Model file for the job. Use its own axes, mm. A direction names the side the tool comes from. Give positions to 0.01 mm unless a question says otherwise; leave off trailing zeros. Loops run counter-clockwise (first coordinate to the right, second up) from the corner with the lowest first, then second, coordinate; pieces in that order, holes last. Notation, with made-up numbers: M 66.5,37 L 76.5,37 A21 ccw 76.5,49 Z; hole C 17.25,25.5 d7. An arc over 180 degrees is marked long. Use CSV: the item, a comma, the result in double quotes. Start each with the question number.
(1) Slice it at C-C on y = 6. State how many separate pieces and enclosed holes the cut face has, and give its area (3 significant figures).
(2) Slice it at B-B on x = 102.5. List the corners of the cut face in (y, z).
(3) Tool access for faces 3 (the face through (-140, 6, 289.5)), 4 (the face through (-2, 6, 337.5)): list every direction of +Z, -Z, +X, -X, +Y, -Y with a clear straight run to the whole face (end or side of a thin tool).
(4) Two-plate mould, pull along X, no slides. Class faces 1 (the face through (72, 6, -6)), 2 (the face through (-24, 12, -2)): pulls with the +X half, pulls with the -X half, needs draft (parallel to the pull), parting line crosses it, or undercut.
(5) Wall check: line 1 along Z through (x, y) = (-47, 7.5); line 2 along X through (y, z) = (8.75, -297.5); line 3 along X through (y, z) = (9, 129). Give the ranges that are in metal, low to high. Write a range as from..to.
(6) Slice it at A-A on z = -281. List the corners of the cut face in (x, y), and give its area (3 significant figures).
```python
from build123d import *

# Parameters (mm, degrees)
SKETCH1_W               = 310
SKETCH1_H               = 675
SKETCH1_W_2             = 300
SKETCH1_H_2             = 665
SKETCH1_W_3             = 260
SKETCH1_H_3             = 625
SKETCH1_W_4             = 250
SKETCH1_H_4             = 615
BOSS_EXTRUDE1_DEPTH     = 12
SKETCH2_W               = 12
SKETCH2_H               = 12
CUT_EXTRUDE1_DEPTH      = 1
CUT_EXTRUDE1_DEPTH_BACK = 13
SKETCH3_W               = 105
SKETCH3_H               = 12
BOSS_EXTRUDE2_DEPTH     = 12


with BuildPart() as part:
    # Sketch1 → Boss-Extrude1 (new body)
    with BuildSketch(Plane(origin=(0, 0, 0), x_dir=(1, 0, 0), z_dir=(0, 1, 0))):
        Rectangle(SKETCH1_W, SKETCH1_H)
        Rectangle(SKETCH1_W_2, SKETCH1_H_2, mode=Mode.SUBTRACT)
        Rectangle(SKETCH1_W_2, SKETCH1_H_2)
        Rectangle(SKETCH1_W_3, SKETCH1_H_3, mode=Mode.SUBTRACT)
        Rectangle(SKETCH1_W_3, SKETCH1_H_3)
        Rectangle(SKETCH1_W_4, SKETCH1_H_4, mode=Mode.SUBTRACT)
    extrude(amount=BOSS_EXTRUDE1_DEPTH)

    # Sketch2 → Cut-Extrude1 (cut, two sides)
    with BuildSketch(Plane(origin=(0, 12, 0), x_dir=(1, 0, 0), z_dir=(0, 1, 0))) as cut_extrude1_sk:
        with Locations((-140, -295.5)):
            Rectangle(SKETCH2_W, SKETCH2_H)
        with Locations((-140, 295.5)):
            Rectangle(SKETCH2_W, SKETCH2_H)
        with Locations((140, 295.5)):
            Rectangle(SKETCH2_W, SKETCH2_H)
        with Locations((140, -295.5)):
            Rectangle(SKETCH2_W, SKETCH2_H)
    extrude(amount=CUT_EXTRUDE1_DEPTH, mode=Mode.SUBTRACT)
    extrude(cut_extrude1_sk.sketch, amount=-CUT_EXTRUDE1_DEPTH_BACK, mode=Mode.SUBTRACT)

    # Sketch3 → Boss-Extrude2 (add)
    with BuildSketch(Plane(origin=(0, 12, 0), x_dir=(1, 0, 0), z_dir=(0, 1, 0))):
        with Locations((-72.5, 0)):
            Rectangle(SKETCH3_W, SKETCH3_H)
        with Locations((72.5, 0)):
            Rectangle(SKETCH3_W, SKETCH3_H)
    extrude(amount=-BOSS_EXTRUDE2_DEPTH)


solid = part.part
```
Reply:
1,separate pieces,"1"
1,enclosed holes,"5"
1,area,"57,400 mm^2"
2,outline,"M 0,-337.5 L 12,-337.5 L 12,-307.5 L 0,-307.5 Z; M 0,-6 L 12,-6 L 12,6 L 0,6 Z; M 0,307.5 L 12,307.5 L 12,337.5 L 0,337.5 Z"
3,face 3,"+Y, -Y"
3,face 4,"+Z, +X, -X, +Y, -Y"
4,face 1,"undercut"
4,face 2,"needs draft"
5,line 1,"z = -337.5..-307.5, -6..6, 307.5..337.5"
5,line 2,"x = -155..-146, -134..-125, 125..134, 146..155"
5,line 3,"x = -155..-125, 125..155"
6,outline,"M -155,0 L -125,0 L -125,12 L -155,12 Z; M 125,0 L 155,0 L 155,12 L 125,12 Z"
6,area,"720 mm^2"
